Source: CAD feature listing. Evaluate the final solid. Frame: model axes, mm. Face numbers are marked on the shaded views. A direction names the side the tool comes from. Give positions to 0.01 mm unless a question says otherwise; leave off trailing zeros. Write each loop counter-clockwise with the first axis right and the second up, starting at its lowest first coordinate (ties: lowest second). Pieces come first, ordered by that corner, then holes. Notation, with made-up numbers: (-5, -2) -> (31, -2) arc R20 cw to (31, 35) -> close; hole circle Ø9 at (-23, 21.5). An arc over 180 degrees is marked (long way). Write item = value, one per line.
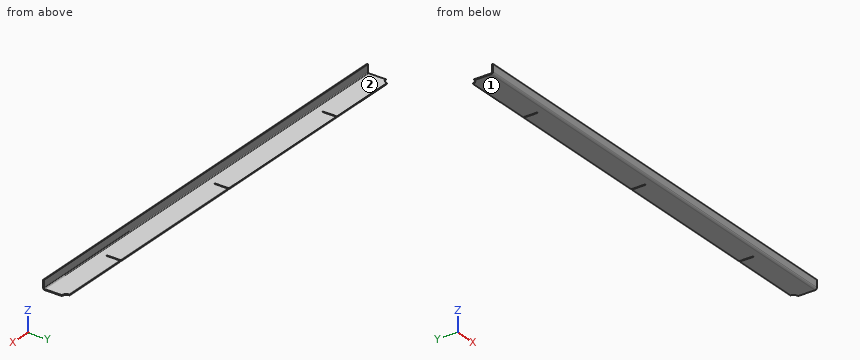
Autodesk Inventor part; units mm, degrees
ref_plane "YZ Plane" through (0, 0, 0) normal (1, 0, 0) x (0, 1, 0)
ref_plane "XZ Plane" through (0, 0, 0) normal (0, 1, 0) x (-1, 0, 0)
ref_plane "XY Plane" through (0, 0, 0) normal (0, 0, 1) x (1, 0, 0)
sketch "Sketch1" plane through (0, 0, 0) normal (0, 0, 1) x (1, 0, 0)
  line L0 (-750, 78.1594) -> (750, 78.1594)
  line L1 (750, 78.1594) -> (750, 0)
  line L2 (750, 0) -> (-750, 0)
  line L3 (-750, 0) -> (-750, 78.1594)
  point P0 (0, 0)
  point P1 (0, 0)
  dimension "d0" = 1500
  dimension "d1" = 78.1594
extrude "Plate1" add sketch "Sketch1" along normal blind 3
sketch "Sketch2" plane through (750, 3, 0) normal (0, -1, 0) x (1, 0, 0)
  line L0 (-1500, 0) -> (0, 0)
  line L1 (0, 0) -> (0, 30)
  line L2 (0, 30) -> (-1500, 30)
  line L3 (-1500, 30) -> (-1500, 0)
edge flange "Flange1" height 30 angle 90 thickness 3 bend radius 3 thickness toward (0, -1, 0) relief tear relief width 3 relief depth 1.5 edges at (0, 0, 3) wall of the first edge with corners at (-750, 3, 0) (750, 3, 0) (750, 3, 30) (-750, 3, 30)
bend "Bend1"
corner "Corner1"
sketch "Sketch5" plane through (0, 0, 0) normal (0, 0, -1) x (-1, 0, 0)
  line L0 (750, 78.1594) -> (-750, 78.1594)
  line L1 (500, 78.1594) -> (500, 31)
  line L2 (500, 31) -> (503, 31)
  line L3 (503, 31) -> (503, 78.1594)
  line L4 (750, 0) -> (-750, 0)
  point P0 (0, 0)
  dimension "d18" = 3
  dimension "d19" = 247
  dimension "d20" = 31
extrude "Extrusion1" cut sketch "Sketch5" against normal through all
pattern_linear "Rectangular Pattern1" count 3 spacing 500 along (1, 0, 0) of "Extrusion1"
sketch "Sketch6" plane through (0, 0, 0) normal (0, 0, -1) x (-1, 0, 0)
  line L0 (-750, 78.1594) -> (-750, 6)
  circle A0 centre (-750, 78.1594) radius 15
  line L1 (-750, 78.1594) -> (-500, 78.1594)
  point P0 (0, 0)
  point P1 (-735, 78.1594)
  point P2 (-750, 63.1594)
  dimension "d24" = 30
extrude "Extrusion2" cut sketch "Sketch6" against normal through all contours L1 A0 L0 picked at (-740.1254, 77.0468)
mirror "Mirror1" about plane through (0, 0, 0) normal (1, 0, 0) of "Extrusion2"
equation "\"d1\" = Стрингер_6"
equation "\"d18\" = Thickness"
equation "\"d2\" = Thickness"
equation "\"d3\" = BendReliefWidth"
equation "\"d4\" = BendReliefDepth"
equation "\"d5\" = MinimumRemnant"
equation "\"d6\" = TransitionRadius"
equation "\"d9\" = BendRadius"
equation "\"d10\" = CornerReliefSize"
equation "\"d11\" = GapSize"
equation "\"d12\" = JacobiRadiusSize"
equation "\"BendRadius\" = Thickness"
equation "\"BendReliefWidth\" = Thickness"
equation "\"BendReliefDepth\" = 0.5 * Thickness"
equation "\"CornerReliefSize\" = 4 * Thickness"
equation "\"MinimumRemnant\" = 2 * Thickness"
equation "\"TransitionRadius\" = BendRadius"
equation "\"JacobiRadiusSize\" = BendRadius"
equation "\"GapSize\" = Thickness"
properties part number "МОО 056 стрингер борт 61"
(1) Section query B-B (x = -527). Return loops of the section in (y, z), plus the area to 3 significant figures.
Values follow:
outline = (0, 6) arc R6 ccw to (6, 0) -> (78.16, 0) -> (78.16, 3) -> (6, 3) arc R3 cw to (3, 6) -> (3, 30) -> (0, 30) -> close
area = 310 mm2
(2) First-contact query: pin 1 (4 mm diameter, centred on x = -381, y = 10, fed in from +Z); pin 2 (1.5 mm diameter, centred on x = -1.5, z = 1, fed in from +Y). Flat tips, straight axial feed; report the tip coordinate or a pass-through.
Values follow:
pin_1 = 3
pin_2 = 31
(3) Section query C-C (z = 21.5). Return loops of the section in (x, y), plus the area to 3 significant figures.
Values follow:
outline = (-750, 0) -> (750, 0) -> (750, 3) -> (-750, 3) -> close
area = 4,500 mm2
(4) Section query A-A (y = 43.5). Return loops of the section in (x, z).
Values follow:
outline = (-750, 0) -> (-503, 0) -> (-503, 3) -> (-750, 3) -> close; (-500, 0) -> (-3, 0) -> (-3, 3) -> (-500, 3) -> close; (0, 0) -> (497, 0) -> (497, 3) -> (0, 3) -> close; (500, 0) -> (750, 0) -> (750, 3) -> (500, 3) -> close
(5) Access query for the marked faces 1 and 2. Directions: +Z, -Z, +X, -X, +Y, -Y. A direction counts if a zero-diameter tool reaches every point of the face in a straight line with its end or side. Return the directions, or none.
Values follow:
face_1 = -Z, +X, -X, +Y, -Y
face_2 = +Z, +X, -X, +Y
(6) Material intervals for line 1 (Y direction, x = -273.5, z = 14); line 2 (Y direction, x = 312, z = 4.75), sorted ascending.
Values follow:
line_1 = 0 to 3
line_2 = 0.13 to 3.27
